```python
from build123d import *

# Parameters (mm, degrees)
SKETCH1_W           = 36
SKETCH1_H           = 34.5
BOSS_EXTRUDE1_DEPTH = 3
SKETCH2_W           = 36
SKETCH2_H           = 34.5
SKETCH2_W_2         = 30
SKETCH2_H_2         = 28.5
SKETCH2_R           = 1.5
BOSS_EXTRUDE2_DEPTH = 1.8
SKETCH3_W           = 36
SKETCH3_H           = 34.5
SKETCH3_W_2         = 30
SKETCH3_H_2         = 28.5
BOSS_EXTRUDE3_DEPTH = 1.6
CHAMFER1_SIZE       = 1.5
SKETCH5_W           = 12
SKETCH5_H           = 3
BOSS_EXTRUDE4_DEPTH = 15
SKETCH6_R           = 1.6
CUT_EXTRUDE1_DEPTH  = 55.260575006
FILLET1_R           = 6


with BuildPart() as part:
    # Sketch1 → Boss-Extrude1 (new body)
    with BuildSketch(Plane(origin=(0, 0, 0), x_dir=(1, 0, 0), z_dir=(0, 1, 0))):
        with Locations((18, 17.25)):
            Rectangle(SKETCH1_W, SKETCH1_H)
    extrude(amount=BOSS_EXTRUDE1_DEPTH)

    # Sketch2 → Boss-Extrude2 (add)
    # profile 1 of 3: a face of its own
    with BuildSketch(Plane(origin=(0, 3, 0), x_dir=(1, 0, 0), z_dir=(0, 1, 0))):
        with Locations((18, 17.25)):
            Rectangle(SKETCH2_W, SKETCH2_H)
        with Locations((18, 17.25)):
            Rectangle(SKETCH2_W_2, SKETCH2_H_2, mode=Mode.SUBTRACT)
    # profile 2 of 3: a face of its own
    with BuildSketch(Plane(origin=(0, 3, 0), x_dir=(1, 0, 0), z_dir=(0, 1, 0))):
        with Locations(Location((7.3, 9.5, 0), (0, 0, 90))):
            Circle(SKETCH2_R)
    # profile 3 of 3: a face of its own
    with BuildSketch(Plane(origin=(0, 3, 0), x_dir=(1, 0, 0), z_dir=(0, 1, 0))):
        with Locations(Location((28.8, 9.5, 0), (0, 0, 90))):
            Circle(SKETCH2_R)
    extrude(amount=BOSS_EXTRUDE2_DEPTH)

    # Sketch3 → Boss-Extrude3 (add)
    # profile 1 of 5: a face of its own
    with BuildSketch(Plane(origin=(0, 4.8, 0), x_dir=(1, 0, 0), z_dir=(0, 1, 0))):
        with Locations((18, 17.25)):
            Rectangle(SKETCH3_W, SKETCH3_H)
        with Locations((18, 17.25)):
            Rectangle(SKETCH3_W_2, SKETCH3_H_2, mode=Mode.SUBTRACT)
    # profile 2 of 5: a face of its own
    with BuildSketch(Plane(origin=(0, 4.8, 0), x_dir=(1, 0, 0), z_dir=(0, 1, 0))):
        with BuildLine():
            ThreePointArc((30.784313483, 9.75), (28.8, 11.5), (26.815686517, 9.75))
            Line((26.815686517, 9.75), (30.784313483, 9.75))
        make_face()
    # profile 3 of 5: a face of its own
    with BuildSketch(Plane(origin=(0, 4.8, 0), x_dir=(1, 0, 0), z_dir=(0, 1, 0))):
        with BuildLine():
            ThreePointArc((26.815686517, 9.25), (28.8, 7.5), (30.784313483, 9.25))
            Line((30.784313483, 9.25), (26.815686517, 9.25))
        make_face()
    # profile 4 of 5: a face of its own
    with BuildSketch(Plane(origin=(0, 4.8, 0), x_dir=(1, 0, 0), z_dir=(0, 1, 0))):
        with BuildLine():
            ThreePointArc((9.284313483, 9.75), (7.3, 11.5), (5.315686517, 9.75))
            Line((5.315686517, 9.75), (9.284313483, 9.75))
        make_face()
    # profile 5 of 5: a face of its own
    with BuildSketch(Plane(origin=(0, 4.8, 0), x_dir=(1, 0, 0), z_dir=(0, 1, 0))):
        with BuildLine():
            ThreePointArc((5.315686517, 9.25), (7.3, 7.5), (9.284313483, 9.25))
            Line((9.284313483, 9.25), (5.315686517, 9.25))
        make_face()
    extrude(amount=BOSS_EXTRUDE3_DEPTH)

    # Chamfer1
    chamfer1_edges = [part.edges().sort_by_distance(p)[0] for p in [
        (7.3, 6.4, -11.5),
        (7.3, 6.4, -7.5),
        (28.8, 6.4, -11.5),
        (28.8, 6.4, -7.5),
    ]]
    chamfer(chamfer1_edges, length=CHAMFER1_SIZE)

    # Sketch5 → Boss-Extrude4 (add)
    with BuildSketch(Plane(origin=(0, 6.4, 0), x_dir=(1, 0, 0), z_dir=(0, 1, 0))):
        with Locations((6, 1.5)):
            Rectangle(SKETCH5_W, SKETCH5_H)
        with Locations((30, 1.5)):
            Rectangle(SKETCH5_W, SKETCH5_H)
    extrude(amount=BOSS_EXTRUDE4_DEPTH)

    # Sketch6 → Cut-Extrude1 (cut, through all)
    with BuildSketch(Plane.XY):
        with Locations((5, 16.4)):
            Circle(SKETCH6_R)
        with Locations((31, 16.4)):
            Circle(SKETCH6_R)
    extrude(amount=-CUT_EXTRUDE1_DEPTH, mode=Mode.SUBTRACT)

    # Fillet1
    fillet1_edges = [part.edges().sort_by_distance(p)[0] for p in [
        (1.5, 6.4, -3),
        (34.5, 6.4, -3),
    ]]
    fillet(fillet1_edges, radius=FILLET1_R)


solid = part.part
```
Input: part model. Units: mm. Frame: model coordinates. A direction names the side the tool comes from. Give positions to 0.01 mm unless a question says otherwise; leave off trailing zeros. Loops run counter-clockwise (first coordinate to the right, second up) from the corner with the lowest first, then second, coordinate; pieces in that order, holes last.
1) Section query C-C on z = -26. Return the cut outline in (x, y).
A:
outline: (0, 0) - (36, 0) - (36, 6.4) - (33, 6.4) - (33, 3) - (3, 3) - (3, 6.4) - (0, 6.4) - close
2) Line query: L1, parallel to Y at x = 31, z = -1; L2, parallel to Z at x = 5, y = 5; L3, parallel to Z at x = 32, y = 7.5. Output: solid intervals per line, ascending.
A:
L1: y = 0 to 14.8, 18 to 21.4
L2: z = -34.5 to -31.5, -3 to 0
L3: z = -3 to 0
3) Section query B-B on y = 16.4. Return the cut outline in (x, z), and give its area (3 significant figures).
A:
outline: (0, -3) - (3.4, -3) - (3.4, 0) - (0, 0) - close; (6.6, -3) - (12, -3) - (12, 0) - (6.6, 0) - close; (24, -3) - (29.4, -3) - (29.4, 0) - (24, 0) - close; (32.6, -3) - (36, -3) - (36, 0) - (32.6, 0) - close
area: 52.8 mm2
4) Mould query, pull axis Z, two halves, no side actions, for faces 1 (the flat face through (18, 6, 0)), 2 (the flat face through (29, 5, -9.25)), 3 (the cylindrical face through (29.73, 15.43, -1.48)). Classes: released by +Z, released by -Z, zero draft, split by the parting line, or undercut.
A:
face 1: released by +Z
face 2: undercut
face 3: zero draft
5) Reachability of faces 4 (the flat face through (12, 14, -1)), 5 (the flat face through (3, 6, -16)), 6 (the cylindrical face through (30.264, 3.887, -9.175)) from +Z, -Z, +X, -X, +Y, -Y: full face, straight path, thin tool, end or side. Return the list, or none.
A:
face 4: +Z, -Z, +Y
face 5: +Y
face 6: none
6) Section query A-A on y = 13.75. Return the cut outline in (x, z), and give its area (3 significant figures).
A:
outline: (0, -3) - (12, -3) - (12, 0) - (0, 0) - close; (24, -3) - (36, -3) - (36, 0) - (24, 0) - close
area: 72.0 mm2
7) Contact query for flat-ended pins moving along their axis: pin 1 (4.5 mm diameter, centred on y = 10, z = -20.5, fed in from +X); pin 2 (1 mm diameter, centred on x = 5.5, z = -27, fed in from +Y); pin 3 (5 mm diameter, centred on x = 5.5, y = 15.5, fed in from -Z). Output: stop coordinate, or through.
A:
pin 1: passes through
pin 2: stops at y = 3
pin 3: stops at z = -3
8) Section query D-D on x = 12.5. Return the cut outline in (y, z).
A:
outline: (0, -34.5) - (6.4, -34.5) - (6.4, -31.5) - (3, -31.5) - (3, -3) - (6.4, -3) - (6.4, 0) - (0, 0) - close
